Autodesk Inventor part; units mm, degrees
ref_plane "YZ Plane" through (0, 0, 0) normal (1, 0, 0) x (0, 1, 0)
ref_plane "XZ Plane" through (0, 0, 0) normal (0, 1, 0) x (-1, 0, 0)
ref_plane "XY Plane" through (0, 0, 0) normal (0, 0, 1) x (1, 0, 0)
sketch "스케치1" plane through (0, 0, 0) normal (0, 1, 0) x (-1, 0, 0)
  line L0 (10, 26) -> (-10, 26)
  line L1 (-10, 26) -> (-10, -26)
  line L2 (-10, -26) -> (10, -26)
  line L3 (10, -26) -> (10, 26)
  line L4 (10, 26) -> (-10, -26) construction
  line L5 (-10, 26) -> (10, -26) construction
  line L6 (6, 22) -> (-6, 22)
  line L7 (-6, 22) -> (-6, -22)
  line L8 (-6, -22) -> (6, -22)
  line L9 (6, -22) -> (6, 22)
  line L10 (7.75, 10.5) -> (-7.75, 10.5)
  line L11 (-7.75, 10.5) -> (-7.75, -10.5) construction
  line L12 (-7.75, -10.5) -> (7.75, -10.5)
  line L13 (7.75, -10.5) -> (7.75, 10.5) construction
  line L14 (7.75, 10.5) -> (-7.75, -10.5) construction
  line L15 (-7.75, 10.5) -> (7.75, -10.5) construction
  line L16 (6, 14.5) -> (-6, 14.5)
  line L17 (0, 0) -> (3.5234, 0)
  line L18 (6, -14.5) -> (-6, -14.5)
  point P0 (0, 10.5)
  point P1 (-6, 10.5)
  point P2 (6, 10.5)
  point P3 (6, -10.5)
  point P4 (-6, -10.5)
  dimension "d0" = 20
  dimension "d1" = 52
  dimension "d2" = 4
  dimension "d3" = 15.5
  dimension "d4" = 21
  dimension "d5" = 4
extrude "돌출1" add sketch "스케치1" along normal blind 5 contours L3 L2 L1 L0 | L9 L10 L7 L16 | L9 L18 L7 L12
sketch "스케치2" plane through (0, 5, 0) normal (0, 1, 0) x (1, 0, 0)
  circle A0 centre (0, -12.5) radius 1
  line L0 (0, 0) -> (-3.3387, 0)
  line L1 (6, -10.5) -> (-6, -10.5)
  circle A1 centre (0, 12.5) radius 1
  dimension "d8" = 2
  dimension "d9" = 2
hole "구멍1" at (0, 5, 12.5) at (0, 5, -12.5) direction (0, -1, 0) diameter 2 end through all countersink diameter 3 countersink angle 90
sketch "스케치3" plane through (10, 0, 26) normal (1, 0, 0) x (0, 0, -1)
  line L0 (0, 0) -> (1.3, -10)
  line L1 (1.3, -10) -> (4.3, -10)
  line L2 (4.3, -10) -> (2.9721, 0.2144)
  line L3 (0, 0) -> (52, 0)
  line L4 (26, 0) -> (26, -7.8)
  line L5 (52, 0) -> (50.7, -10)
  line L6 (50.7, -10) -> (47.7, -10)
  line L7 (47.7, -10) -> (49.0279, 0.2144)
  point P0 (49, 0)
  point P1 (3, 0)
  dimension "d17" = 10
  dimension "d18" = 4.3
  dimension "d19" = 3
extrude "돌출2" add sketch "스케치3" against normal up to surface (20 mm away)
fillet "모깎기1" radius 2 2 edges at (0, 5, 26) (0, 5, -26)
properties part number "스텝모터 상판"
Work out the finished part from the listing and answer in its coordinate system (mm). A direction names the side the tool comes from. Round coordinates to 2 decimals unless told otherwise and drop trailing zeros. Write each loop counter-clockwise with the first axis right and the second up, starting at its lowest first coordinate (ties: lowest second). Pieces come first, ordered by that corner, then holes. Notation, with made-up numbers: (-18.75, 69.5) - (29.25, 69.5) arc R24 cw to (29.25, 88.5) - close; hole circle Ø1 at (5.5, 51.25). An arc over 180 degrees is marked (long way). Answer in a Markdown table with one row per item. Add a question column.
1. Find the intervals of material crossed by line 1 along Z through (x, y) = (0, 2.65); line 2 along X through (y, z) = (3, 21.5); line 3 along X through (y, z) = (1.75, -12.5), in increasing order. Write a range as from..to.
2. A cutting plane is placed at C-C, the plane z = -1. Determine the outline of the cut face in (x, y), and give its area (3 significant figures).
3. Given pin 1 (10 mm diameter, centred on x = -2, z = -9, fed in from -Y); pin 2 (2.5 mm diameter, centred on x = 0, z = 12.5, fed in from +Y), each flat-ended and moving along its own axis, determine where each tip first touches the part or whether it passes through.
4. A cutting plane is placed at D-D, the plane y = 2.5. Determine the outline of the cut face in (x, z), and give its area (3 significant figures).
5. A cutting plane is placed at B-B, the plane x = -4.5. Determine the outline of the cut face in (y, z).
6. For faces 4 (the flat face through (0, 2, -22)), 5 (the flat face through (0, 2, -14.5)), 6 (the flat face through (0.14, -5.07, -22.34)), 7 (the flat face through (0, 1, -26)), 8 (the flat face through (7, 5, 0)), determine the directions among +Z, -Z, +X, -X, +Y, -Y from which every point of the face is accessible in a straight line to the end or side of a thin tool.
7. A cutting plane is placed at A-A, the plane y = -7. Determine the outline of the cut face in (x, z).
8. The mould has two halves that part along X. Classify faces 1 (the flat face through (0.14, -4.93, 25.36)), 2 (the flat face through (0, 2, 14.5)), 3 (the flat face through (-10, 1, 0)): +X half, -X half, draft (parallel to the pull), parting line (faces both ways), or undercut.
Worked out:
| question | item | result |
|---|---|---|
| 1 | line 1 | -26..-22, -14.5..-13.5, -11.5..-10.5, 10.5..11.5, 13.5..14.5, 22..26 |
| 1 | line 2 | -10..-6, 6..10 |
| 1 | line 3 | -10..-1, 1..10 |
| 2 | outline | (-10, 0) - (-6, 0) - (-6, 5) - (-10, 5) - close; (6, 0) - (10, 0) - (10, 5) - (6, 5) - close |
| 2 | area | 40.0 mm^2 |
| 3 | pin 1 | y = 0 |
| 3 | pin 2 | y = 4.75 |
| 4 | outline | (-10, -26) - (10, -26) - (10, 26) - (-10, 26) - close; hole (-6, -22) - (6, -22) - (6, -14.5) - (-6, -14.5) - close; hole (-6, -10.5) - (6, -10.5) - (6, 10.5) - (-6, 10.5) - close; hole (-6, 14.5) - (6, 14.5) - (6, 22) - (-6, 22) - close; hole circle Ø2 at (0, -12.5); hole circle Ø2 at (0, 12.5) |
| 4 | area | 602 mm^2 |
| 5 | outline | (-10, -24.7) - (0, -26) - (3, -26) arc R2 ccw to (5, -24) - (5, -22) - (0, -22) - (0, -23) - (-10, -21.7) - close; (-10, 21.7) - (0, 23) - (0, 22) - (5, 22) - (5, 24) arc R2 ccw to (3, 26) - (0, 26) - (-10, 24.7) - close; (0, -14.5) - (5, -14.5) - (5, -10.5) - (0, -10.5) - close; (0, 10.5) - (5, 10.5) - (5, 14.5) - (0, 14.5) - close |
| 6 | face 4 | +Y |
| 6 | face 5 | +Y, -Y |
| 6 | face 6 | +X, -X |
| 6 | face 7 | -Z, +X, -X, +Y, -Y |
| 6 | face 8 | +Z, -Z, +X, -X, +Y |
| 7 | outline | (-10, -25.09) - (10, -25.09) - (10, -22.09) - (-10, -22.09) - close; (-10, 22.09) - (10, 22.09) - (10, 25.09) - (-10, 25.09) - close |
| 8 | face 1 | draft |
| 8 | face 2 | undercut |
| 8 | face 3 | -X half |
